Could you check a few things on this model? Use its own coordinates, in mm. Face numbers are marked on the shaded views. A direction names the side the tool comes from. Round coordinates to 2 decimals unless told otherwise and drop trailing zeros. Write each loop counter-clockwise with the first axis right and the second up, starting at its lowest first coordinate (ties: lowest second). Pieces come first, ordered by that corner, then holes. Notation, with made-up numbers: (43, 4.25) -> (60, 4.25) arc R19 ccw to (60, 16.25) -> close; hole circle Ø3 at (-22.5, 4). An arc over 180 degrees is marked (long way). Return JSON: item names as keys, results as strings.
from build123d import *

# Parameters (mm, degrees)
BOSS_EXTRUDE1_DEPTH     = 3
SKETCH2_R               = 2.625
BOSS_EXTRUDE2_DEPTH     = 4
SKETCH3_W               = 9
SKETCH3_H               = 3
CUT_EXTRUDE1_DEPTH      = 46.717380795
CUT_EXTRUDE2_DEPTH      = 47.391760164
CUT_EXTRUDE2_DEPTH_BACK = 47.391760164
SKETCH4_R               = 0.625
CUT_EXTRUDE3_DEPTH      = 33.475581638
CUT_EXTRUDE3_DEPTH_BACK = 33.475581638
SKETCH5_R               = 0.625
CUT_EXTRUDE4_DEPTH      = 34.635958629
CUT_EXTRUDE4_DEPTH_BACK = 34.635958629
SKETCH6_R               = 0.625
BOSS_EXTRUDE3_DEPTH     = 25
SCALE1_SCALE            = 1.3


with BuildPart() as part:
    # Sketch1 → Boss-Extrude1 (new body)
    with BuildSketch(Plane(origin=(0, 0, 0), x_dir=(1, 0, 0), z_dir=(0, 1, 0))):
        with BuildLine():
            Line((6.591682084, 11.417128277), (15, 25.980762114))
            ThreePointArc((15, 25.980762114), (16.768876635, 25.128389411), (18.644755802, 24.548267761))
            Line((18.644755802, 24.548267761), (19.091682084, 26.497692522))
            Line((19.091682084, 26.497692522), (24.091682084, 26.497692522))
            Line((24.091682084, 26.497692522), (24.538608366, 24.548267761))
            ThreePointArc((24.538608366, 24.548267761), (26.414487532, 25.128389411), (28.183364168, 25.980762114))
            Line((28.183364168, 25.980762114), (36.591682084, 11.417128277))
            ThreePointArc((36.591682084, 11.417128277), (34.969067352, 10.311422526), (33.528727683, 8.976924338))
            Line((33.528727683, 8.976924338), (34.993515908, 7.615162444))
            Line((34.993515908, 7.615162444), (32.493515908, 3.285035425))
            Line((32.493515908, 3.285035425), (30.581801401, 3.872698291))
            ThreePointArc((30.581801401, 3.872698291), (30.146261903, 1.958078454), (30, 0))
            Line((30, 0), (13.183364168, 0))
            ThreePointArc((13.183364168, 0), (13.037102264, 1.958078454), (12.601562767, 3.872698291))
            Line((12.601562767, 3.872698291), (10.68984826, 3.285035425))
            Line((10.68984826, 3.285035425), (8.18984826, 7.615162444))
            Line((8.18984826, 7.615162444), (9.654636485, 8.976924338))
            ThreePointArc((9.654636485, 8.976924338), (8.214296816, 10.311422526), (6.591682084, 11.417128277))
        make_face()
    extrude(amount=BOSS_EXTRUDE1_DEPTH)

    # Sketch2 → Boss-Extrude2 (add)
    with BuildSketch(Plane(origin=(0, 3, 0), x_dir=(1, 0, 0), z_dir=(0, 1, 0))):
        with Locations(Location((21.591682084, 12.465963463, 0), (0, 0, 90))):
            Circle(SKETCH2_R)
    extrude(amount=BOSS_EXTRUDE2_DEPTH)

    # Sketch3 → Cut-Extrude1 (cut, through all)
    with BuildSketch(Plane.XZ):
        with Locations((21.591682084, -1.5)):
            Rectangle(SKETCH3_W, SKETCH3_H)
        Polygon((8.545841042, -14.801830878), (13.045841042, -22.596059512), (15.643917253, -21.096059512), (11.143917253, -13.301830878), align=None)
        Polygon((34.637523126, -14.801830878), (32.039446914, -13.301830878), (27.539446914, -21.096059512), (30.137523126, -22.596059512), align=None)
    extrude(amount=-CUT_EXTRUDE1_DEPTH, mode=Mode.SUBTRACT)

    # Sketch4 → Cut-Extrude2 (cut, two sides: drawn at the far end of the back side and taken through both)
    with BuildSketch(Plane(origin=(2.25, 0, 3.897114317), x_dir=(-0.8660254037844389, 0, 0.4999999999999997), z_dir=(-0.4999999999999997, 0, -0.8660254037844389)).offset(-CUT_EXTRUDE2_DEPTH_BACK)):
        with Locations((-35.89789039, 1.5)):
            Circle(SKETCH4_R)
    extrude(amount=CUT_EXTRUDE2_DEPTH + CUT_EXTRUDE2_DEPTH_BACK, mode=Mode.SUBTRACT)

    # Sketch5 → Cut-Extrude3 (cut, two sides: drawn at the far end of the back side and taken through both)
    with BuildSketch(Plane(origin=(8.545841042, 0, -14.801830878), x_dir=(-0.8660254037844383, 0, -0.5000000000000008), z_dir=(0.5000000000000007, 0, -0.8660254037844382)).offset(-CUT_EXTRUDE3_DEPTH_BACK)):
        with Locations((-1.5, 1.5)):
            Circle(SKETCH5_R)
    extrude(amount=CUT_EXTRUDE3_DEPTH + CUT_EXTRUDE3_DEPTH_BACK, mode=Mode.SUBTRACT)

    # Sketch6 → Cut-Extrude4 (cut, two sides: drawn at the far end of the back side and taken through both)
    with BuildSketch(Plane.ZY.offset(-26.091682084).offset(-CUT_EXTRUDE4_DEPTH_BACK)):
        with Locations((-1.5, 1.5)):
            Circle(SKETCH6_R)
    extrude(amount=CUT_EXTRUDE4_DEPTH + CUT_EXTRUDE4_DEPTH_BACK, mode=Mode.SUBTRACT)

    # Sketch7 → Boss-Extrude3 (add)
    with BuildSketch(Plane(origin=(0, 3, 0), x_dir=(1, 0, 0), z_dir=(0, 1, 0))):
        with BuildLine():
            Line((8.18984826, 7.615162444), (10.68984826, 3.285035425))
            Line((10.68984826, 3.285035425), (12.12363414, 3.725782575))
            ThreePointArc((12.12363414, 3.725782575), (10.983890093, 6.341551902), (9.288439429, 8.636483864))
            Line((9.288439429, 8.636483864), (8.18984826, 7.615162444))
        make_face()
        with BuildLine():
            Line((32.493515908, 3.285035425), (34.993515908, 7.615162444))
            Line((34.993515908, 7.615162444), (33.894924739, 8.636483864))
            ThreePointArc((33.894924739, 8.636483864), (32.199474075, 6.341551902), (31.059730028, 3.725782575))
            Line((31.059730028, 3.725782575), (32.493515908, 3.285035425))
        make_face()
        with BuildLine():
            Line((19.091682084, 26.497692522), (24.091682084, 26.497692522))
            Line((24.091682084, 26.497692522), (24.426876795, 25.035623951))
            ThreePointArc((24.426876795, 25.035623951), (21.591682084, 24.714786587), (18.756487372, 25.035623951))
            Line((18.756487372, 25.035623951), (19.091682084, 26.497692522))
        make_face()
    extrude(amount=BOSS_EXTRUDE3_DEPTH)


with BuildPart() as part_1:
    # Scale1: scaled about (21.591676284, 5.938563321, -12.465985005)
    add(part.part.scale(SCALE1_SCALE).moved(Location((-6.477502885, -1.781568996, 3.739795502))))


solid = part_1.part
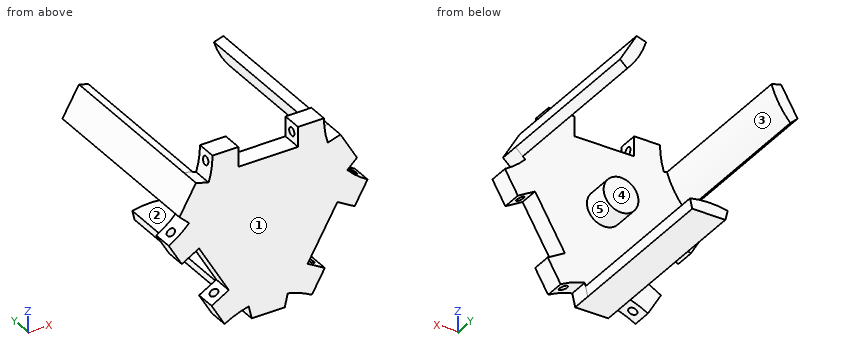
1) If I drill on probe 1 along Y at (x, z) = (29, -8); probe 2 along Y at (x, z) = (24.5, -14); probe 3 along Z at (x, y) = (8, 19.5), over which ranges is the centre line in solid material (lowest first)? Write a range as [from, to].
Return value:
{"probe 1": "[-1.78, 2.12]", "probe 2": "[-1.78, 7.32]", "probe 3": "[-4.15, -0.71]"}
2) I want a section at D-D, the plane x = 16.5. Please give me the cut outline in (y, z), and give its area (3 significant figures).
Return value:
{"outline": "(-1.78, -28.51) -> (2.12, -28.51) -> (2.12, -0.16) -> (-1.78, -0.16) -> close", "area": "111 mm²"}
3) I want a section at B-B, the plane x = 22.5. Please give me the cut outline in (y, z).
Return value:
{"outline": "(-1.78, -30.71) -> (34.62, -30.71) -> (34.62, -28.41) -> (2.12, -28.41) -> (2.12, -15.76) -> (7.32, -15.76) -> (7.32, -9.18) -> (2.12, -9.18) -> (2.12, -0.16) -> (-1.78, -0.16) -> close"}
4) Will these pins go through, and if not, where does the flat tip stop? pin 1 Ø5 at (x, z) = (28, -21.5) entering from +Y; pin 2 Ø2 at (y, z) = (-1, 2.5) entering from -X; pin 3 Ø1.2 at (y, z) = (1, 2) entering from +X; pin 4 Ø1.5 at (x, z) = (8.5, -17) entering from -Y.
Return value:
{"pin 1": "y = 2.12", "pin 2": "x = 10.51", "pin 3": "x = 32.68", "pin 4": "through"}
5) I want a section at C-C, the plane z = -3.5. Please give me the cut outline in (x, y) (3 decimals), and give its area (3 significant figures).
Return value:
{"outline": "(5.705, -1.782) -> (37.478, -1.782) -> (37.478, 34.618) -> (34.847, 34.618) -> (34.847, 2.118) -> (8.336, 2.118) -> (8.336, 34.618) -> (5.705, 34.618) -> close", "area": "295 mm²"}
6) I want a section at A-A, the plane y = 26.5. Please give me the cut outline in (x, z).
Return value:
{"outline": "(4.17, -6.16) -> (5.6, -7.49) arc R16.49 ccw to (9.28, -1.1) -> (7.42, -0.53) -> close; (17.91, -28.81) -> (18.34, -30.71) -> (24.84, -30.71) -> (25.28, -28.81) arc R16.49 ccw to start; (33.9, -1.1) arc R16.49 ccw to (37.59, -7.49) -> (39.01, -6.16) -> (35.76, -0.53) -> close"}
7) Thinking about a two-plate mould opening in Z: for the marked faces 3, 4 and 5, which applies, pulls with the +Z half, pulls with the -Z half, needs draft (parallel to the pull), parting line crosses it, or undercut?
Return value:
{"face 3": "pulls with the -Z half", "face 4": "needs draft", "face 5": "undercut"}
8) For the marked faces 1 and 2, which set-ups out of +Z, -Z, +X, -X, +Y, -Y let a thin tool reach every point of the face, with its end or its side?
Return value:
{"face 1": "+Z, -Z, +X, -X, -Y", "face 2": "+Y"}
